Verification items for the finished model (mm, model axes). A direction names the side the tool comes from. Coordinates: 2 decimals unless noted, no trailing zeros. Order: outer loops, then holes, each group sorted by start corner. A loop starts at its lowest first (then second) coordinate and runs counter-clockwise, first axis right, second up. Notation, with made-up numbers: M -30.75,77.5 L 15.25,77.5 A31 ccw 15.25,102.5 Z; hole C 77,-23.5 d8. An arc over 180 degrees is marked long. Return JSON: item names as keys, results as strings. Group by question number.
1. Section check A-A, the plane z = 11.5. Record the cut outline in (x, y), plus the area to 3 significant figures.
2. Mould release check, pull along X, two halves, no side actions. Record for faces 1 (the cylindrical face through (-1.281, -34.576, 12.254)), 2 (the flat face through (11, 33.67, 4)), 3 (the flat face through (-12.329, 36.778, 9.988)): +X half, -X half, draft (parallel to the pull), parting line (faces both ways), or undercut.
3. Set-up check for faces 4 (the cylindrical face through (-28.948, 9.116, 3.186)), 5 (the flat face through (16, 25, 2.2)), 6 (the cylindrical face through (14.72, 30.77, 3.02)): record each of +Z, -Z, +X, -X, +Y, -Y from which the full face is reachable in a straight line by a thin tool's end or side.
4. Material ranges on line 1 along Y through (x, z) = (0, 5.75); line 2 along X through (y, z) = (11.5, 6.5); line 3 along Y through (x, z) = (0, 4.5), recorded low to high.
5. Gauge pin test, flat ends, axial feed: pin 1 (2 mm diameter, centred on x = -4.5, z = 6.5, fed in from -Y); pin 2 (4 mm diameter, centred on x = 14, z = 5, fed in from +Y); pin 3 (6 mm diameter, centred on x = -3, y = 12.5, fed in from -Z). Record the tip position at first contact, or that the pin passes through.
```python
from build123d import *

# Parameters (mm, degrees)
F3_DEPTH      = 15
F4_R          = 30.35
F5_DEPTH      = 12
F8_DEPTH      = 5.2
F9_T1_DEPTH   = 15
F9_T6_DEPTH   = 27.1954073321
F9_S7_R       = 32.6
F9_T8_DEPTH   = 16
F9_S9_R       = 34.6
F9_T10_DEPTH  = 16
F9_T14_DEPTH  = 27.1954073321
F9_S15_R      = 32.6
F9_T16_DEPTH  = 16
F9_S17_R      = 34.6
F9_T18_DEPTH  = 16
F9_T23_DEPTH  = 27.1954073321
F9_S24_R      = 34.6
F9_T25_DEPTH  = 16
F9_T29_DEPTH  = 22.7968974984
F9_T37_DEPTH  = 27.1954073321
F9_S39_R      = 34.6
F9_T40_DEPTH  = 16
F9_T43_DEPTH  = 22.7968974984
F10_SIZE      = 3
F11_T1_DEPTH  = 24.2
F11_T3_DEPTH  = 6.7426406871
F11_T5_DEPTH  = 6.7426406871
F11_T7_DEPTH  = 1.6807325889
F11_T10_ANGLE = 303.1497240065
F11_T12_ANGLE = 61.5748620049
F11_T14_ANGLE = 61.5748620049


# Not quite as in the source:
# - a fillet or chamfer that OpenCascade refuses, or shapes differently, is made with other operations: its cross-section is extruded or revolved along the edge and cut away or added


with BuildPart() as f1:
    # F0 (on Front) → F1 (revolve)
    with BuildSketch(Plane.XZ):
        Polygon((-30.35, 1.2), (-30.35, 0), (-28.35, 0), (-28.35, 18.2), (0, 18.2), (0, 20.2), (-30.35, 20.2), (-32.6, 20.2), (-32.6, 8.2), (-30.35, 8.2), (-30.35, 5.2), (-29.35, 5.2), (-29.35, 4.2), (-30.35, 4.2), (-30.35, 2.2), (-29.35, 2.2), (-29.35, 1.2), align=None)
    revolve(axis=Axis((0, 0, 19.2), (0, 0, -1)))

    # F2 (on face) → F3 (join)
    with BuildSketch(Plane.XY.offset(20.2)):
        with BuildLine():
            Line((-13.85, 38.2565491622), (-13.85, 31.707057574))
            ThreePointArc((-13.85, 31.707057574), (0, -34.6), (13.85, 31.707057574))
            Line((13.85, 31.707057574), (13.85, 38.2565491622))
            Line((13.85, 38.2565491622), (-13.85, 38.2565491622))
        make_face()
        with BuildLine():
            ThreePointArc((11.85, 30.3700098782), (0, -32.6), (-11.85, 30.3700098782))
            Line((-11.85, 30.3700098782), (-11.85, 33.6700098782))
            Line((-11.85, 33.6700098782), (-9.35, 33.6700098782))
            Line((-9.35, 33.6700098782), (-9.35, 31.2303938496))
            ThreePointArc((-9.35, 31.2303938496), (0, 32.6), (9.35, 31.2303938496))
            Line((9.35, 31.2303938496), (9.35, 33.6700098782))
            Line((9.35, 33.6700098782), (11.85, 33.6700098782))
            Line((11.85, 33.6700098782), (11.85, 30.3700098782))
        make_face(mode=Mode.SUBTRACT)
    extrude(amount=-F3_DEPTH)

    # F4 (on face) → F5 (join)
    with BuildSketch(Plane(origin=(0, 0, 8.2), x_dir=(1, 0, 0), z_dir=(0, 0, -1))):
        with BuildLine():
            ThreePointArc((13.85, -31.707057574), (0, 34.6), (-13.85, -31.707057574))
            Line((-13.85, -31.707057574), (-13.85, -38.2565491622))
            Line((-13.85, -38.2565491622), (13.85, -38.2565491622))
            Line((13.85, -38.2565491622), (13.85, -31.707057574))
        make_face()
        Circle(F4_R, mode=Mode.SUBTRACT)
    extrude(amount=-F5_DEPTH)

    # F7 (on face) → F8 (join, through all)
    with BuildSketch(Plane(origin=(0, 0, 5.2), x_dir=(1, 0, 0), z_dir=(0, 0, -1))):
        with BuildLine():
            Line((-13.85, -29.5116502419), (-13.85, -38.2565491622))
            Line((-13.85, -38.2565491622), (13.85, -38.2565491622))
            Line((13.85, -38.2565491622), (13.85, -29.5116502419))
            ThreePointArc((13.85, -29.5116502419), (12.8571651353, -29.9575250093), (11.85, -30.3700098782))
            Line((11.85, -30.3700098782), (11.85, -33.6700098782))
            Line((11.85, -33.6700098782), (9.35, -33.6700098782))
            Line((9.35, -33.6700098782), (9.35, -31.2303938496))
            ThreePointArc((9.35, -31.2303938496), (0, -32.6), (-9.35, -31.2303938496))
            Line((-9.35, -31.2303938496), (-9.35, -33.6700098782))
            Line((-9.35, -33.6700098782), (-11.85, -33.6700098782))
            Line((-11.85, -33.6700098782), (-11.85, -30.3700098782))
            ThreePointArc((-11.85, -30.3700098782), (-12.8571651353, -29.9575250093), (-13.85, -29.5116502419))
        make_face()
    extrude(amount=F8_DEPTH)

    # F9: fillet of radius 5 on 4 edges, made by hand

    # F9_s2 → F9_t1 (join)
    with BuildSketch(Plane.XY.offset(5.2)):
        with BuildLine():
            ThreePointArc((-16.4699494949, 30.4286175111), (-14.5546389834, 32.2665444625), (-13.85, 34.8258165733))
            Line((-13.85, 34.8258165733), (-13.85, 31.707057574))
            ThreePointArc((-13.85, 31.707057574), (-15.1734451129, 31.0954428077), (-16.4699494949, 30.4286175111))
        make_face()
        with BuildLine():
            ThreePointArc((16.4699494949, 30.4286175111), (14.5546389834, 32.2665444625), (13.85, 34.8258165733))
            Line((13.85, 34.8258165733), (13.85, 31.707057574))
            ThreePointArc((13.85, 31.707057574), (15.1734451129, 31.0954428077), (16.4699494949, 30.4286175111))
        make_face()
    extrude(amount=F9_T1_DEPTH)


with BuildPart() as f9_tool4:
    # F9_s5 → F9_t6 (new body)
    with BuildSketch(Plane.XZ.offset(-44.207057574)):
        with BuildLine():
            ThreePointArc((13.85, 0.2), (15.3144660941, 3.7355339059), (18.85, 5.2))
            Line((18.85, 5.2), (13.85, 5.2))
            Line((13.85, 5.2), (13.85, 0.2))
        make_face()
    extrude(amount=F9_T6_DEPTH)

    # F9_s7 → F9_t8 (cut, symmetric)
    with BuildSketch(Plane.XY.offset(2.7)):
        Circle(F9_S7_R)
    extrude(amount=F9_T8_DEPTH, both=True, mode=Mode.SUBTRACT)

    # F9_s9 → F9_t10 (intersect, symmetric)
    with BuildSketch(Plane.XY.offset(2.7)):
        Circle(F9_S9_R)
    extrude(amount=F9_T10_DEPTH, both=True, mode=Mode.INTERSECT)


with BuildPart() as f1_1:
    add(f1.part)

    # F9_t3: union F9_tool4
    add(f9_tool4.part)


with BuildPart() as f9_tool12:
    # F9_s13 → F9_t14 (new body)
    with BuildSketch(Plane.XZ.offset(-17.0116502419)):
        with BuildLine():
            ThreePointArc((-18.85, 5.2), (-15.3144660941, 3.7355339059), (-13.85, 0.2))
            Line((-13.85, 0.2), (-13.85, 5.2))
            Line((-13.85, 5.2), (-18.85, 5.2))
        make_face()
    extrude(amount=-F9_T14_DEPTH)

    # F9_s15 → F9_t16 (cut, symmetric)
    with BuildSketch(Plane.XY.offset(2.7)):
        Circle(F9_S15_R)
    extrude(amount=F9_T16_DEPTH, both=True, mode=Mode.SUBTRACT)

    # F9_s17 → F9_t18 (intersect, symmetric)
    with BuildSketch(Plane.XY.offset(2.7)):
        Circle(F9_S17_R)
    extrude(amount=F9_T18_DEPTH, both=True, mode=Mode.INTERSECT)


with BuildPart() as f1_2:
    add(f1_1.part)

    # F9_t11: union F9_tool12
    add(f9_tool12.part)


with BuildPart() as f9_tool21:
    # F9_s22 → F9_t23 (new body)
    with BuildSketch(Plane.XZ.offset(-17.0116502419)):
        with BuildLine():
            ThreePointArc((-18.85, 5.2), (-15.3144660941, 3.7355339059), (-13.85, 0.2))
            Line((-13.85, 0.2), (-13.85, 5.2))
            Line((-13.85, 5.2), (-18.85, 5.2))
        make_face()
    extrude(amount=-F9_T23_DEPTH)

    # F9_s24 → F9_t25 (cut, symmetric)
    with BuildSketch(Plane.XY.offset(2.7)):
        Circle(F9_S24_R)
    extrude(amount=F9_T25_DEPTH, both=True, mode=Mode.SUBTRACT)

    split(bisect_by=Plane.XZ.offset(-38.2565491622), keep=Keep.TOP)


with BuildPart() as f9_tool27:
    # F9_s28 → F9_t29 (new body)
    with BuildSketch(Plane.XY.offset(-2.5968974984)):
        with BuildLine():
            ThreePointArc((-16.4699494949, 30.4286175111), (-14.5546389834, 32.2665444625), (-13.85, 34.8258165733))
            Line((-13.85, 34.8258165733), (-13.85, 31.707057574))
            ThreePointArc((-13.85, 31.707057574), (-15.1734451129, 31.0954428077), (-16.4699494949, 30.4286175111))
        make_face()
    extrude(amount=F9_T29_DEPTH)

    split(bisect_by=Plane.XY, keep=Keep.TOP)

    split(bisect_by=Plane.XY.offset(5.2), keep=Keep.BOTTOM)


with BuildPart() as f9_tool21_1:
    add(f9_tool21.part)

    # F9_t32: intersect F9_tool27
    add(f9_tool27.part, mode=Mode.INTERSECT)


with BuildPart() as f1_3:
    add(f1_2.part)

    # F9_t19: union F9_tool21
    add(f9_tool21_1.part)


with BuildPart() as f9_tool35:
    # F9_s36 → F9_t37 (new body)
    with BuildSketch(Plane.XZ.offset(-44.207057574)):
        with BuildLine():
            ThreePointArc((13.85, 0.2), (15.3144660941, 3.7355339059), (18.85, 5.2))
            Line((18.85, 5.2), (13.85, 5.2))
            Line((13.85, 5.2), (13.85, 0.2))
        make_face()
    extrude(amount=F9_T37_DEPTH)

    split(bisect_by=Plane.XZ.offset(-38.2565491622), keep=Keep.TOP)

    # F9_s39 → F9_t40 (cut, symmetric)
    with BuildSketch(Plane.XY.offset(2.7)):
        Circle(F9_S39_R)
    extrude(amount=F9_T40_DEPTH, both=True, mode=Mode.SUBTRACT)


with BuildPart() as f9_tool41:
    # F9_s42 → F9_t43 (new body)
    with BuildSketch(Plane.XY.offset(20.2)):
        with BuildLine():
            ThreePointArc((16.4699494949, 30.4286175111), (14.5546389834, 32.2665444625), (13.85, 34.8258165733))
            Line((13.85, 34.8258165733), (13.85, 31.707057574))
            ThreePointArc((13.85, 31.707057574), (15.1734451129, 31.0954428077), (16.4699494949, 30.4286175111))
        make_face()
    extrude(amount=-F9_T43_DEPTH)

    split(bisect_by=Plane.XY, keep=Keep.TOP)

    split(bisect_by=Plane.XY.offset(5.2), keep=Keep.BOTTOM)


with BuildPart() as f9_tool35_1:
    add(f9_tool35.part)

    # F9_t46: intersect F9_tool41
    add(f9_tool41.part, mode=Mode.INTERSECT)


with BuildPart() as f1_4:
    add(f1_3.part)

    # F9_t33: union F9_tool35
    add(f9_tool35_1.part)

    # F10
    f10_edges = [f1_4.edges().sort_by_distance(p)[0] for p in [
        (13.85, 38.256549, 12.7),
        (13.85, 38.256549, 2.6),
        (-13.85, 38.256549, 12.7),
        (-13.85, 38.256549, 2.6),
    ]]
    chamfer(f10_edges, length=F10_SIZE)

    # F11: fillet of radius 0.5 on 8 edges, made by hand

    # F11_s2 → F11_t1 (cut)
    with BuildSketch(Plane.YZ.offset(-12.1)):
        with BuildLine():
            ThreePointArc((38.2565491622, 19.7), (38.1101025528, 20.0535533906), (37.7565491622, 20.2))
            Line((37.7565491622, 20.2), (38.2565491622, 20.2))
            Line((38.2565491622, 20.2), (38.2565491622, 19.7))
        make_face()
    extrude(amount=F11_T1_DEPTH, mode=Mode.SUBTRACT)

    # F11_s4 → F11_t3 (cut)
    with BuildSketch(Plane(origin=(9.8193911046, 9.8193911046, 0), x_dir=(0, 0, 1), z_dir=(0.7071067812, 0.7071067812, 0))):
        with BuildLine():
            ThreePointArc((19.7, -34.7235739133), (20.0535533906, -34.5771273039), (20.2, -34.2235739133))
            Line((20.2, -34.2235739133), (20.2, -34.7235739133))
            Line((20.2, -34.7235739133), (19.7, -34.7235739133))
        make_face()
    extrude(amount=F11_T3_DEPTH, mode=Mode.SUBTRACT)

    # F11_s6 → F11_t5 (cut)
    with BuildSketch(Plane(origin=(-14.5871580576, 14.5871580576, 0), x_dir=(0, 0, 1), z_dir=(0.7071067812, -0.7071067812, 0))):
        with BuildLine():
            ThreePointArc((19.7, -34.7235739133), (20.0535533906, -34.5771273039), (20.2, -34.2235739133))
            Line((20.2, -34.2235739133), (20.2, -34.7235739133))
            Line((20.2, -34.7235739133), (19.7, -34.7235739133))
        make_face()
    extrude(amount=F11_T5_DEPTH, mode=Mode.SUBTRACT)

    # F11_s8 → F11_t7 (cut)
    with BuildSketch(Plane.XZ.offset(-36.5065491622)):
        with BuildLine():
            ThreePointArc((-13.85, 19.7), (-13.7035533906, 20.0535533906), (-13.35, 20.2))
            Line((-13.35, 20.2), (-13.85, 20.2))
            Line((-13.85, 20.2), (-13.85, 19.7))
        make_face()
        with BuildLine():
            ThreePointArc((13.85, 19.7), (13.7035533906, 20.0535533906), (13.35, 20.2))
            Line((13.35, 20.2), (13.85, 20.2))
            Line((13.85, 20.2), (13.85, 19.7))
        make_face()
    extrude(amount=F11_T7_DEPTH, mode=Mode.SUBTRACT)

    # F11_s9 → F11_t10 (revolve, cut)
    with BuildSketch(Plane(origin=(0, 0, 0), x_dir=(0, 0, 1), z_dir=(0.8794398125, 0.476010101, 0))):
        with BuildLine():
            ThreePointArc((20.2, -34.1), (20.0535533906, -34.4535533906), (19.7, -34.6))
            Line((19.7, -34.6), (20.2, -34.6))
            Line((20.2, -34.6), (20.2, -34.1))
        make_face()
    revolve(axis=Axis((0, 0, 20.2), (0, 0, 1)), revolution_arc=F11_T10_ANGLE, mode=Mode.SUBTRACT)

    # F11_s11 → F11_t12 (revolve, cut)
    with BuildSketch(Plane(origin=(-4e-10, -2e-10, 0), x_dir=(0, 0, 1), z_dir=(-0.8794398125, -0.476010101, 0))):
        with BuildLine():
            ThreePointArc((19.7, 34.6), (20.0535533906, 34.4535533906), (20.2, 34.1))
            Line((20.2, 34.1), (20.2, 34.6))
            Line((20.2, 34.6), (19.7, 34.6))
        make_face()
    revolve(axis=Axis((-18.8499999998, 34.8258165732, 20.2), (0, 0, 1)), revolution_arc=F11_T12_ANGLE, mode=Mode.SUBTRACT)

    # F11_s13 → F11_t14 (revolve, cut)
    with BuildSketch(Plane(origin=(4e-10, -2e-10, 0), x_dir=(0, 0, 1), z_dir=(0.8794398125, -0.476010101, 0))):
        with BuildLine():
            ThreePointArc((19.7, -34.6), (20.0535533906, -34.4535533906), (20.2, -34.1))
            Line((20.2, -34.1), (20.2, -34.6))
            Line((20.2, -34.6), (19.7, -34.6))
        make_face()
    revolve(axis=Axis((18.8499999998, 34.8258165732, 20.2), (0, 0, -1)), revolution_arc=F11_T14_ANGLE, mode=Mode.SUBTRACT)


solid = f1_4.part
```
Answers follow:
{
 "1": {"outline": "M -16.47,30.43 A34.6 ccw long 16.47,30.43 A5 cw 13.85,34.83 L 13.85,35.26 L 10.85,38.26 L -10.85,38.26 L -13.85,35.26 L -13.85,34.83 A5 cw Z; hole C 0,0 d56.7", "area": "1,360 mm^2"},
 "2": {"face 1": "parting line", "face 2": "undercut", "face 3": "-X half"},
 "3": {"face 4": "-Z", "face 5": "none", "face 6": "-Z, +X, +Y"},
 "4": {"line 1": "-34.6 to -32.6, -30.35 to -28.35, 28.35 to 30.35, 32.6 to 38.26", "line 2": "-32.63 to -30.5, -28.09 to -25.91, 25.91 to 28.09, 30.5 to 32.63", "line 3": "-29.35 to -28.35, 28.35 to 29.35, 32.6 to 38.26"},
 "5": {"pin 1": "y = -34.42", "pin 2": "y = 37.11", "pin 3": "z = 18.2"}
}
